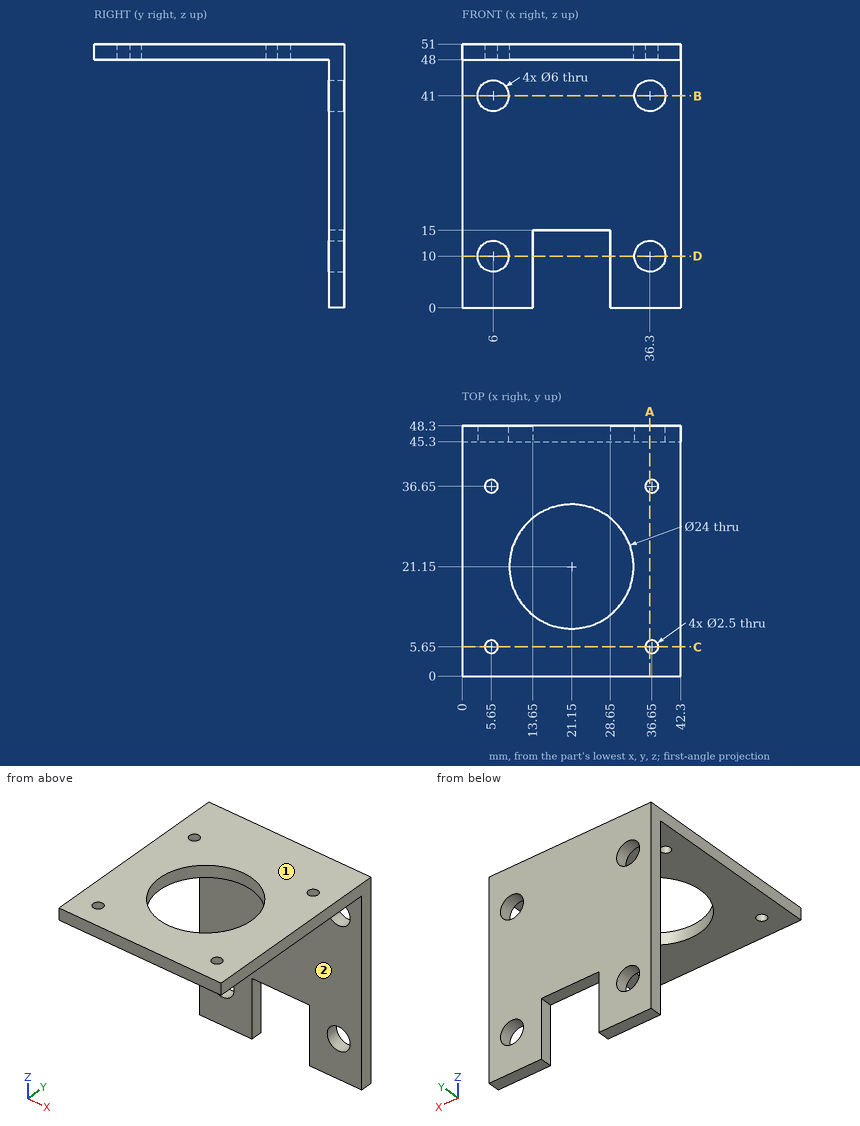
Check sheet for the drawn part. Datum: minimum x, y, z corner. Units: mm. A direction names the side the tool comes from. Coordinates: 2 decimals unless noted, no trailing zeros. Loops run counter-clockwise (first coordinate to the right, second up) from the corner with the lowest first, then second, coordinate; pieces in that order, holes last. Notation, with made-up numbers: (15.5, -10.5) -> (36.5, -10.5) arc R23 cw to (36.5, -1.5) -> close; hole circle Ø2 at (89, 31.5). An arc over 180 degrees is marked (long way). Answer in a Markdown table with one row per item.
1) Access from +Z, -Z, +X, -X, +Y, -Y to the whole of each face (thin tool, end or side, straight path). Record for the marked faces 1 and 2.
The answers:
| item | result |
|---|---|
| face 1 | +Z, +X, -X, +Y, -Y |
| face 2 | -Z, +X, -X, -Y |
2) Scan lines: line 1 along Z through (x, y) = (6, 46.85); line 2 along Z through (x, y) = (32.5, 4); line 3 along Y through (x, z) = (3, 25). Record each from-to range of solid material in increasing order. Write a range as from..to.
The answers:
| item | result |
|---|---|
| line 1 | z = 0..7, 13..38, 44..51 |
| line 2 | z = 48..51 |
| line 3 | y = 45.3..48.3 |
3) Section check A-A (x = 36.3). Record the cut outline in (y, z), and give its area (4 significant figures).
The answers:
| item | result |
|---|---|
| outline | (0, 48) -> (4.45, 48) -> (4.45, 51) -> (0, 51) -> close; (6.85, 48) -> (35.45, 48) -> (35.45, 51) -> (6.85, 51) -> close; (37.85, 48) -> (45.3, 48) -> (45.3, 44) -> (48.3, 44) -> (48.3, 51) -> (37.85, 51) -> close; (45.3, 0) -> (48.3, 0) -> (48.3, 7) -> (45.3, 7) -> close; (45.3, 13) -> (48.3, 13) -> (48.3, 38) -> (45.3, 38) -> close |
| area | 238.5 mm2 |
4) Section check D-D (z = 10). Record the cut outline in (x, y), and give its area (3 significant figures).
The answers:
| item | result |
|---|---|
| outline | (0, 45.3) -> (3, 45.3) -> (3, 48.3) -> (0, 48.3) -> close; (9, 45.3) -> (13.65, 45.3) -> (13.65, 48.3) -> (9, 48.3) -> close; (28.65, 45.3) -> (33.3, 45.3) -> (33.3, 48.3) -> (28.65, 48.3) -> close; (39.3, 45.3) -> (42.3, 45.3) -> (42.3, 48.3) -> (39.3, 48.3) -> close |
| area | 45.9 mm2 |
5) Section check B-B (z = 41). Record the cut outline in (x, y).
The answers:
| item | result |
|---|---|
| outline | (0, 45.3) -> (3, 45.3) -> (3, 48.3) -> (0, 48.3) -> close; (9, 45.3) -> (33.3, 45.3) -> (33.3, 48.3) -> (9, 48.3) -> close; (39.3, 45.3) -> (42.3, 45.3) -> (42.3, 48.3) -> (39.3, 48.3) -> close |
6) Depth check by flat-ended pin: P1, Ø12.5, axis at x = 25, z = 33, coming from the -Y side; P2, Ø0.9, axis at x = 24, y = 47, coming from the -Z side; P3, Ø4, axis at x = 36.65, y = 5.65, coming from the -Z side. Enter the tip coordinate at first touch or a pass-through.
The answers:
| item | result |
|---|---|
| P1 | stops at y = 45.3 |
| P2 | stops at z = 15 |
| P3 | stops at z = 48 |
7) Section check C-C (y = 5.65). Record the cut outline in (x, z).
The answers:
| item | result |
|---|---|
| outline | (0, 48) -> (4.4, 48) -> (4.4, 51) -> (0, 51) -> close; (6.9, 48) -> (35.4, 48) -> (35.4, 51) -> (6.9, 51) -> close; (37.9, 48) -> (42.3, 48) -> (42.3, 51) -> (37.9, 51) -> close |
